Read the model definition and answer for the solid it produces. Units are mm, in the model's axes. Face numbers are marked on the shaded views. Round coordinates to 2 decimals unless told otherwise and drop trailing zeros. Write each loop counter-clockwise with the first axis right and the second up, starting at its lowest first coordinate (ties: lowest second). Pieces come first, ordered by that corner, then holes. Notation, with made-up numbers: (59.5, -10.75) - (107.5, -10.75) arc R27 cw to (107.5, 12.25) - close; hole circle Ø1 at (-14, 52.5). An arc over 180 degrees is marked (long way). One line per item, written item: value. Start each with the question number.
(1) The mould has two halves that part along Z. Classify the marked faces 1, 2 and 3: +Z half, -Z half, draft (parallel to the pull), parting line (faces both ways), or undercut.
(2) A cutting plane is placed at B-B, the plane x = 0. Determine the outline of the cut face in (y, z).
(3) A cutting plane is placed at D-D, the plane z = 30.5. State how many separate pieces and enclosed holes the cut face has, plus the area to 3 significant figures.
(4) A cutting plane is placed at C-C, the plane y = 5. Determine the outline of the cut face in (x, z).
(5) A cutting plane is placed at A-A, the plane z = 0. Determine the outline of the cut face in (x, y), plus the area to 3 significant figures.
(6) Find the intervals of material crossed by L1, parallel to Z at x = -30.5, y = 2; L2, parallel to Z at x = 0, y = 19; L3, parallel to X at y = 2, z = -30, in increasing order.
(7) Flat-ended cylindrical pins translate along their axes: pin 1 Ø12 at (x, y) = (-12.5, 23.5) entering from +Z; pin 2 Ø3.5 at (x, z) = (30.5, -30.5) entering from +Y; pin 3 Ø12 at (x, y) = (-15.5, 18.5) entering from +Z; pin 4 Ø8 at (x, y) = (20.5, 15) entering from +Z. Find the tip coordinate at first contact, or state that the pin passes through.
from build123d import *

# Parameters (mm, degrees)
SKETCH1_W                                  = 70
SKETCH1_H                                  = 70
BOSS_EXTRUDE1_DEPTH                        = 3
SKETCH2_R                                  = 18
CUT_EXTRUDE1_DEPTH                         = 3
SKETCH3_R                                  = 22
SKETCH3_R_2                                = 19.65
BOSS_EXTRUDE2_DEPTH                        = 30
FILLET1_R                                  = 10
SKETCH4_R                                  = 2.25
CUT_EXTRUDE2_DEPTH                         = 3
MIRROR1_AT_THE_SECOND_PLANE_COPY_1_SKETC_R = 2.25
MIRROR1_AT_THE_SECOND_PLANE_COPY_1_DEPTH   = 3
FILLET4_R                                  = 1


with BuildPart() as part:
    # Sketch1 → Boss-Extrude1 (new body)
    with BuildSketch(Plane(origin=(0, 0, 0), x_dir=(1, 0, 0), z_dir=(0, 1, 0))):
        Rectangle(SKETCH1_W, SKETCH1_H)
    extrude(amount=BOSS_EXTRUDE1_DEPTH)

    # Sketch2 → Cut-Extrude1 (cut)
    with BuildSketch(Plane(origin=(0, 3, 0), x_dir=(1, 0, 0), z_dir=(0, 1, 0))):
        Circle(SKETCH2_R)
    extrude(amount=-CUT_EXTRUDE1_DEPTH, mode=Mode.SUBTRACT)

    # Sketch3 → Boss-Extrude2 (add)
    with BuildSketch(Plane(origin=(0, 3, 0), x_dir=(1, 0, 0), z_dir=(0, 1, 0))):
        Circle(SKETCH3_R)
        Circle(SKETCH3_R_2, mode=Mode.SUBTRACT)
    extrude(amount=BOSS_EXTRUDE2_DEPTH)

    # Fillet1
    fillet1_edges = [part.edges().sort_by_distance(p)[0] for p in [
        (-22, 3, 0),
    ]]
    fillet(fillet1_edges, radius=FILLET1_R)

    # Sketch4 → Cut-Extrude2 (cut)
    with BuildSketch(Plane(origin=(0, 0, 0), x_dir=(-1, 0, 0), z_dir=(0, -1, 0))):
        with Locations((30.5, -30.5)):
            Circle(SKETCH4_R)
    cut_extrude2 = extrude(amount=-CUT_EXTRUDE2_DEPTH, mode=Mode.SUBTRACT)

    # Mirror1: Cut-Extrude2 across plane
    add(cut_extrude2.mirror(Plane(origin=(0, 0, 0), x_dir=(0, 0, 1), z_dir=(1, 0, 0))), mode=Mode.SUBTRACT)

    # Mirror1 at the second plane: Cut-Extrude2 across plane
    add(cut_extrude2.mirror(Plane.XY), mode=Mode.SUBTRACT)

    # Mirror1 at the second plane copy 1 sketc → Mirror1 at the second plane copy 1 (cut)
    with BuildSketch(Plane.XZ):
        with Locations((30.5, -30.5)):
            Circle(MIRROR1_AT_THE_SECOND_PLANE_COPY_1_SKETC_R)
    extrude(amount=-MIRROR1_AT_THE_SECOND_PLANE_COPY_1_DEPTH, mode=Mode.SUBTRACT)

    # Fillet4
    fillet4_edges = [part.edges().sort_by_distance(p)[0] for p in [
        (0, 0, 35),
        (-35, 0, 0),
        (0, 0, -35),
        (35, 0, 0),
    ]]
    fillet(fillet4_edges, radius=FILLET4_R)


solid = part.part
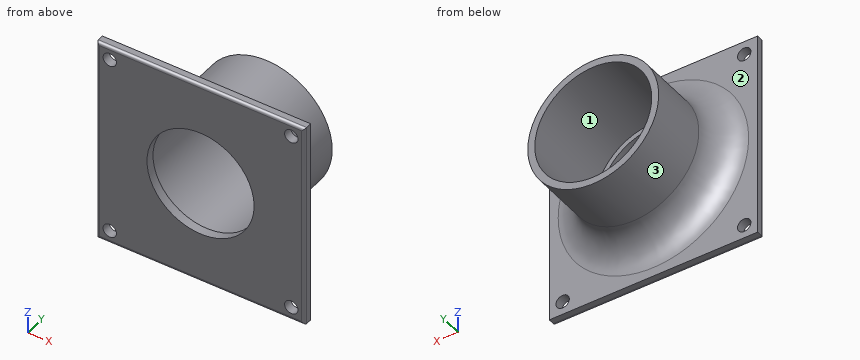
Here are the results:
1. face 1: undercut
1. face 2: draft
1. face 3: parting line
2. outline: (0, -34) arc R1 ccw to (1, -35) - (3, -35) - (3, -32) arc R10 cw to (13, -22) - (33, -22) - (33, -19.65) - (3, -19.65) - (3, -18) - (0, -18) - close; (0, 18) - (3, 18) - (3, 19.65) - (33, 19.65) - (33, 22) - (13, 22) arc R10 cw to (3, 32) - (3, 35) - (1, 35) arc R1 ccw to (0, 34) - close
3. separate pieces: 3
3. enclosed holes: 0
3. area: 184 mm²
4. outline: circle Ø52 at (0, 0); hole circle Ø39.3 at (0, 0)
5. outline: (-35, 1) arc R1 ccw to (-34, 0) - (-18, 0) - (-18, 3) - (-19.65, 3) - (-19.65, 33) - (-22, 33) - (-22, 13) arc R10 cw to (-32, 3) - (-35, 3) - close; (18, 0) - (34, 0) arc R1 ccw to (35, 1) - (35, 3) - (32, 3) arc R10 cw to (22, 13) - (22, 33) - (19.65, 33) - (19.65, 3) - (18, 3) - close
5. area: 285 mm²
6. L1: -35 to -32.75, -28.25 to 28.25, 32.75 to 35
6. L2: -22 to -19.65, 19.65 to 22
6. L3: -35 to -32.69, -28.31 to 28.31, 32.69 to 35
7. pin 1: z = 21.02
7. pin 2: through
7. pin 3: z = 19.84
7. pin 4: z = 14.55
